```python
from build123d import *

# Parameters (mm, degrees)
CYLINDER_R     = 2
CYLINDER_DEPTH = 10
BOX003_W       = 10
BOX003_H       = 11
BOX003_DEPTH   = 13
BOX002_W       = 16
BOX002_H       = 10
BOX002_DEPTH   = 13
BOX001_W       = 44
BOX001_H       = 44
BOX001_DEPTH   = 29
BOX_W          = 50
BOX_H          = 50
BOX_DEPTH      = 31


with BuildPart() as cylinder:
    # Cylinder → Cylinder (new body)
    with BuildSketch(Plane(origin=(6, 6, -1), x_dir=(1, 0, 0), z_dir=(0, 0, 1))):
        Circle(CYLINDER_R)
    extrude(amount=CYLINDER_DEPTH)


with BuildPart() as cylinder001:
    # Link001 base: copy of Cylinder
    add(cylinder.part)


with BuildPart() as cylinder001_1:
    # Link001 placement: moved
    add(cylinder001.part.moved(Location((37, 37, 0))))


with BuildPart() as cube003:
    # Box003 → Box003 (new body)
    with BuildSketch(Plane(origin=(-3, 13, 3), x_dir=(1, 0, 0), z_dir=(0, 0, 1))):
        with Locations((5, 5.5)):
            Rectangle(BOX003_W, BOX003_H)
    extrude(amount=BOX003_DEPTH)


with BuildPart() as cube004:
    # Link base: copy of Cube003
    add(cube003.part)


with BuildPart() as cube004_1:
    # Link placement: moved
    add(cube004.part.moved(Location((47, 0, 0))))


with BuildPart() as cube002:
    # Box002 → Box002 (new body)
    with BuildSketch(Plane(origin=(9, -7, 3), x_dir=(1, 0, 0), z_dir=(0, 0, 1))):
        with Locations((8, 5)):
            Rectangle(BOX002_W, BOX002_H)
    extrude(amount=BOX002_DEPTH)


with BuildPart() as cube001:
    # Box001 → Box001 (new body)
    with BuildSketch(Plane(origin=(3, 3, 3), x_dir=(1, 0, 0), z_dir=(0, 0, 1))):
        with Locations((22, 22)):
            Rectangle(BOX001_W, BOX001_H)
    extrude(amount=BOX001_DEPTH)


with BuildPart() as cut005:
    # Box → Box (new body)
    with BuildSketch(Plane.XY):
        with Locations((25, 25)):
            Rectangle(BOX_W, BOX_H)
    extrude(amount=BOX_DEPTH)

    # Cut: cut Cube001
    add(cube001.part, mode=Mode.SUBTRACT)

    # Cut001: cut Cube002
    add(cube002.part, mode=Mode.SUBTRACT)

    # Cut002: cut Cube003
    add(cube003.part, mode=Mode.SUBTRACT)

    # Cut003: cut Cube004
    add(cube004_1.part, mode=Mode.SUBTRACT)

    # Cut004: cut Cylinder
    add(cylinder.part, mode=Mode.SUBTRACT)

    # Cut005: cut Cylinder001
    add(cylinder001_1.part, mode=Mode.SUBTRACT)


solid = cut005.part
```
Geometry: final body of the model. Coordinates: model frame, mm. A direction names the side the tool comes from. Coordinates: 2 decimals unless noted, no trailing zeros. Order: outer loops, then holes, each group sorted by start corner. A loop starts at its lowest first (then second) coordinate and runs counter-clockwise, first axis right, second up. Notation, with made-up numbers: (33.25, 78) -> (69.25, 78) arc R4 cw to (69.25, 82) -> close; hole circle Ø6 at (40.5, 10.5). An arc over 180 degrees is marked (long way). Answer in a Markdown table with one row per item.
Item 1: Section D-D on y = 20. Output: boundary loops of the cut face in (x, z), plus the area to 3 significant figures.
Return value:
| item | result |
|---|---|
| outline | (0, 0) -> (50, 0) -> (50, 3) -> (0, 3) -> close; (0, 16) -> (3, 16) -> (3, 31) -> (0, 31) -> close; (47, 16) -> (50, 16) -> (50, 31) -> (47, 31) -> close |
| area | 240 mm² |
Item 2: Ray query, L1, parallel to X at y = 6, z = 0.65; L2, parallel to X at y = 43, z = 0.8. Return the intervals inside material, ascending.
Return value:
| item | result |
|---|---|
| L1 | x = 0 to 4, 8 to 50 |
| L2 | x = 0 to 41, 45 to 50 |
Item 3: Contact query for a flat-ended pin moving along its axis: P1, Ø6, axis at x = 27.5, y = 21, coming from the +Z side. Output: stop coordinate, or through.
Return value:
| item | result |
|---|---|
| P1 | stops at z = 3 |
Item 4: Section B-B on x = 20. Output: boundary loops of the cut face in (y, z).
Return value:
| item | result |
|---|---|
| outline | (0, 0) -> (50, 0) -> (50, 31) -> (47, 31) -> (47, 3) -> (0, 3) -> close; (0, 16) -> (3, 16) -> (3, 31) -> (0, 31) -> close |
Item 5: Access query for faces 1 (the flat face through (25, 1, 9)), 2 (the flat face through (25, 0, 19)), 3 (the flat face through (1, 24, 9)), 4 (the flat face through (25, 3, 20)). Directions: +Z, -Z, +X, -X, +Y, -Y. A direction counts if a zero-diameter tool reaches every point of the face in a straight line with its end or side. Return the directions, or none.
Return value:
| item | result |
|---|---|
| face 1 | -Y |
| face 2 | +Z, -Z, +X, -X, -Y |
| face 3 | +X, -X |
| face 4 | +Z |
Item 6: Section C-C on y = 6. Output: boundary loops of the cut face in (x, z).
Return value:
| item | result |
|---|---|
| outline | (0, 0) -> (4, 0) -> (4, 3) -> (3, 3) -> (3, 31) -> (0, 31) -> close; (8, 0) -> (50, 0) -> (50, 31) -> (47, 31) -> (47, 3) -> (8, 3) -> close |
Item 7: Section A-A on z = 13. Output: boundary loops of the cut face in (x, y), plus the area to 3 significant figures.
Return value:
| item | result |
|---|---|
| outline | (0, 0) -> (9, 0) -> (9, 3) -> (3, 3) -> (3, 13) -> (0, 13) -> close; (0, 24) -> (3, 24) -> (3, 47) -> (47, 47) -> (47, 24) -> (50, 24) -> (50, 50) -> (0, 50) -> close; (25, 0) -> (50, 0) -> (50, 13) -> (47, 13) -> (47, 3) -> (25, 3) -> close |
| area | 450 mm² |
Item 8: Draft query along Z for faces 5 (the flat face through (25, 25, 0)), 6 (the flat face through (48, 19, 16)), 7 (the flat face through (25, 47, 17)). Return one class per face: released by +Z, released by -Z, zero draft, split by the parting line, or undercut.
Return value:
| item | result |
|---|---|
| face 5 | released by -Z |
| face 6 | undercut |
| face 7 | zero draft |
